Geometry check sheet. Reference: drawing and pictorial views, mm from the part's lowest x, y, z. A direction names the side the tool comes from. Coordinates: 2 decimals unless noted, no trailing zeros. Loops run counter-clockwise (first coordinate to the right, second up) from the corner with the lowest first, then second, coordinate; pieces in that order, holes last. Notation, with made-up numbers: (-18.75, -35.75) - (8.25, -35.75) arc R11 ccw to (8.25, -18.75) - close; hole circle Ø5 at (37, -11). An arc over 180 degrees is marked (long way). One line per item, written item: value.
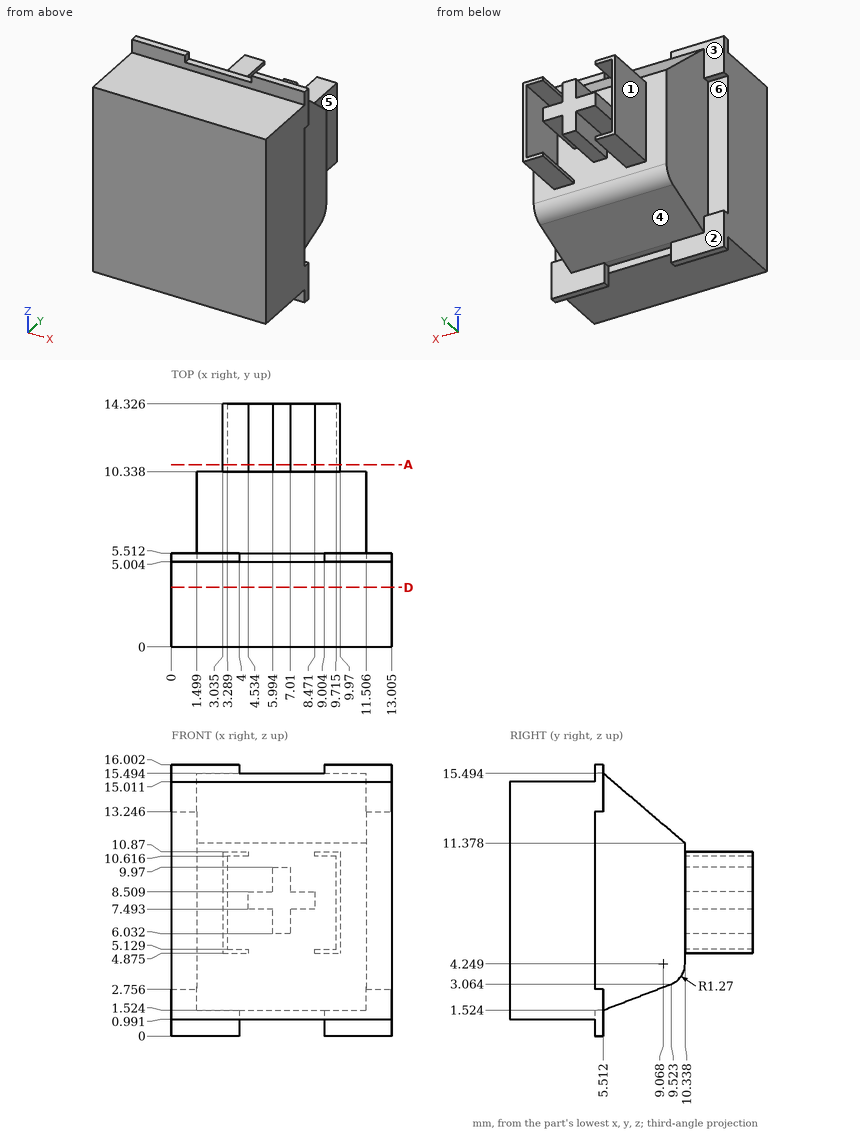
(1) Cross-section at D-D on y = 3.5. Record the cut outline in (x, z) (1 decimal), and give its area (3 significant figures).
Reply:
outline: (0, 1) - (13, 1) - (13, 15) - (0, 15) - close
area: 182 mm2
(2) Material ranges on probe 1 along X at (y, z) = (11.5, 5) (1 decimal); probe 2 along Z at (x, y) = (3.5, 13.5) (1 decimal); probe 3 along X at (y, z) = (8.5, 7), recorded low to high. Write a range as from..to.
Reply:
probe 1: 3..4.5, 8.5..10
probe 2: 4.9..5.1, 10.6..10.9
probe 3: 1.5..11.51
(3) Cross-section at A-A on y = 10.75. State how many separate pieces and enclosed holes the cut face has.
Reply:
separate pieces: 3
enclosed holes: 0
(4) Go/stop test with flat-tipped pins: pin 1 Ø0.7 at (x, y) = (3.5, 13) entering from +Z; pin 2 Ø2 at (x, y) = (6.5, 12.5) entering from +Z; pin 3 Ø1.6 at (x, y) = (4, 13) entering from -Z (1 decimal). Record where each tip stops, or that it passes through.
Reply:
pin 1: z = 10.87
pin 2: z = 9.97
pin 3: z = 4.9
(5) Release check for a two-part mould opening along Z. For the marked faces 4, 5 and 6 record: pulls with the +Z half, pulls with the -Z half, needs draft (parallel to the pull), parting line crosses it, or undercut.
Reply:
face 4: pulls with the -Z half
face 5: needs draft
face 6: undercut
(6) Access from +Z, -Z, +X, -X, +Y, -Y to the whole of each face (thin tool, end or side, straight path). Record for the marked faces 1, 2 and 3.
Reply:
face 1: +Z, -Z, -X, +Y
face 2: -Z, -X, +Y
face 3: +Z, -X, +Y
